Design review of the part built by this model. Coordinates are the model's own, in mm. A direction names the side the tool comes from. Give positions to 0.01 mm unless a question says otherwise; leave off trailing zeros. Loops run counter-clockwise (first coordinate to the right, second up) from the corner with the lowest first, then second, coordinate; pieces in that order, holes last. Notation, with made-up numbers: (-24.75, 24.25) -> (5.25, 24.25) arc R34 cw to (5.25, 57.25) -> close; hole circle Ø7 at (80, -7.75). An arc over 180 degrees is marked (long way). Answer in a Markdown table with one row per item. Add a question column.
(1) For line 1 (Y direction, x = 38, z = 4.5); line 2 (Y direction, x = 38, z = 25); line 3 (Y direction, x = 21, z = 19), list the stretches that pass through material, from the lowest coordinate up.
(2) For pin 1 (12 mm diameter, centred on x = 7, z = 11.5, fed in from -Y); pin 2 (1.5 mm diameter, centred on y = 1.5, z = 14, fed in from +X); pin 3 (5.5 mm diameter, centred on x = 23, z = 1.5, fed in from +Y), all flat-tipped, find the tip position at first contact; note any pin that passes through.
(3) For faces 1 (the flat face through (29, 0, 0)), 2 (the cylindrical face through (42.333, 5.237, 19.297)), 3 (the cylindrical face through (15.72, 5.01, 19.3)), 4 (the flat face through (28.49, 11, 19)), 5 (the flat face through (29, 3.5, 2)), list the 3-axis set-ups (+Z, -Z, +X, -X, +Y, -Y) from which the entire face can be reached by the end or side of a thin tool; tool diameter is ignored.
(4) Consider section C-C on z = 19.5. Write out the cut boundary in (x, y), then the cut area to 3 significant figures.
(5) Draft analysis for pull direction Y (two halves, no side actions). For faces 6 (the cylindrical face through (61.48, -0.08, 2.46)), 7 (the flat face through (29, -3.5, 2)), 8 (the cylindrical face through (55.482, 0.11, 2.465)), state which applies: +Y half, -Y half, draft (parallel to the pull), parting line (faces both ways), or undercut.
(6) Consider section B-B on x = 38. Write out the cut boundary in (y, z), then the cut area to 3 significant figures.
(7) Consider section A-A on y = 0. Write out the cut boundary in (x, z).
(8) Consider section D-D on x = 17.5. Write out the cut boundary in (y, z), then the cut area to 3 significant figures.
from build123d import *

# Parameters (mm, degrees)
SKETCH_R        = 2.5
PAD_DEPTH       = 5
PAD001_DEPTH    = 29
SKETCH002_R     = 1.2
POCKET_DEPTH    = 34.001
SKETCH004_R     = 4.5
POCKET002_DEPTH = 34.001


with BuildPart() as part:
    # Sketch → Pad (new body)
    with BuildSketch(Plane.XY):
        with BuildLine():
            ThreePointArc((0, 3.5), (-3.5, 0), (0, -3.5))
            Line((57.98, -3.5), (0, -3.5))
            ThreePointArc((57.98, -3.5), (61.48, 0), (57.98, 3.5))
            Line((0, 3.5), (57.98, 3.5))
        make_face()
        Circle(SKETCH_R, mode=Mode.SUBTRACT)
        with Locations((57.98, 0)):
            Circle(SKETCH_R, mode=Mode.SUBTRACT)
    extrude(amount=PAD_DEPTH)

    # Sketch001 (on Face8 of Pad) → Pad001 (join)
    with BuildSketch(Plane.XY.offset(5)):
        with BuildLine():
            Line((29.489935, 16), (29.489935, 6))
            Line((28.489935, 6), (29.489935, 6))
            Line((28.489935, 6), (28.489935, 15.99995))
            Line((28.489935, 15.99995), (10.983499, 12.313113))
            ThreePointArc((16.133505, -3.458326), (15.684946, 5.121763), (10.983499, 12.313113))
            Line((16.133505, -3.458326), (41.846495, -3.458326))
            ThreePointArc((46.996509, 12.31312), (42.295055, 5.121768), (41.846495, -3.458326))
            Line((46.996509, 12.31312), (29.489935, 16))
        make_face()
    extrude(amount=PAD001_DEPTH)

    # Sketch002 (on Face18 of Pad001) → Pocket (cut, through all)
    with BuildSketch(Plane.XY.offset(34)):
        with Locations((20, 0)):
            Circle(SKETCH002_R)
        with Locations((38, 0)):
            Circle(SKETCH002_R)
    extrude(amount=-POCKET_DEPTH, mode=Mode.SUBTRACT)

    # Sketch004 → Pocket002 (cut, through all)
    with BuildSketch(Plane.XY.offset(34)):
        with Locations((21, 8)):
            Circle(SKETCH004_R)
        with Locations((37, 8)):
            Circle(SKETCH004_R)
    extrude(amount=-POCKET002_DEPTH, mode=Mode.SUBTRACT)


solid = part.part
Values follow:
| question | item | result |
|---|---|---|
| 1 | line 1 | -3.5 to -1.2, 1.2 to 3.5 |
| 1 | line 2 | -3.46 to -1.2, 1.2 to 3.61, 12.39 to 14.21 |
| 1 | line 3 | -3.46 to -0.66, 0.66 to 3.5, 12.5 to 14.42 |
| 2 | pin 1 | y = 10.16 |
| 2 | pin 2 | x = 41.63 |
| 2 | pin 3 | y = 3.5 |
| 3 | face 1 | -Z, +X, -X, +Y, -Y |
| 3 | face 2 | +Z, +X |
| 3 | face 3 | +Z, -X |
| 3 | face 4 | +Z, -Z, +Y |
| 3 | face 5 | -Z, +X, -X, +Y |
| 4 | outline | (10.98, 12.31) arc R16.5 cw to (16.13, -3.46) -> (41.85, -3.46) arc R16.5 cw to (47, 12.31) -> (29.49, 16) -> (29.49, 6) -> (28.49, 6) -> (28.49, 16) -> close; hole circle Ø9 at (21, 8); hole circle Ø2.4 at (20, 0); hole circle Ø9 at (37, 8); hole circle Ø2.4 at (38, 0) |
| 4 | area | 359 mm2 |
| 5 | face 6 | parting line |
| 5 | face 7 | -Y half |
| 5 | face 8 | undercut |
| 6 | outline | (-3.5, 0) -> (-1.2, 0) -> (-1.2, 34) -> (-3.46, 34) -> (-3.46, 5) -> (-3.5, 5) -> close; (1.2, 0) -> (3.5, 0) -> (3.5, 5) -> (3.61, 5) -> (3.61, 34) -> (1.2, 34) -> close; (12.39, 5) -> (14.21, 5) -> (14.21, 34) -> (12.39, 34) -> close |
| 6 | area | 211 mm2 |
| 7 | outline | (-3.5, 0) -> (-2.5, 0) -> (-2.5, 5) -> (-3.5, 5) -> close; (2.5, 0) -> (18.8, 0) -> (18.8, 34) -> (16.5, 34) -> (16.5, 5) -> (2.5, 5) -> close; (21.2, 0) -> (36.8, 0) -> (36.8, 34) -> (21.2, 34) -> close; (39.2, 0) -> (55.48, 0) -> (55.48, 5) -> (41.48, 5) -> (41.48, 34) -> (39.2, 34) -> close; (60.48, 0) -> (61.48, 0) -> (61.48, 5) -> (60.48, 5) -> close |
| 8 | outline | (-3.5, 0) -> (3.5, 0) -> (3.5, 5) -> (5.17, 5) -> (5.17, 34) -> (-3.46, 34) -> (-3.46, 5) -> (-3.5, 5) -> close; (10.83, 5) -> (13.69, 5) -> (13.69, 34) -> (10.83, 34) -> close |
| 8 | area | 368 mm2 |
